Could you check a few things on this model? Use its own coordinates, in mm. A direction names the side the tool comes from. Round coordinates to 2 decimals unless told otherwise and drop trailing zeros. Write each loop counter-clockwise with the first axis right and the second up, starting at its lowest first coordinate (ties: lowest second). Pieces come first, ordered by that corner, then holes. Notation, with made-up numbers: M 12,73 L 20,73 A23 cw 20,108 Z; hole C 53,-36.75 d8. An arc over 180 degrees is marked long. One line per item, written item: value. Start each with the question number.
(1) I'm going to push a flat-ended pin straight in: pin 1 Ø6 at (x, z) = (12.5, 54) entering from +Y. Where does the tip first touch, or does it pass through?
(2) Thinking about a two-plate mould opening in Z: for faces 4 (the face through (21, 0, 37)), 5 (the face through (21, -3, 72)), 6 (the face through (5, -3, 25)), which applies, released by +Z, released by -Z, zero draft, split by the parting line, or undercut?
(3) If I drill on L1, parallel to Z at x = 21, y = -3.3; L2, parallel to X at y = -3.1, z = 6; L3, parallel to Z at x = 40.5, y = -3.45, over which ranges is the centre line in solid material (lowest first)?
(4) I want a section at B-B on y = -2.2. Please give me the cut outline in (x, z).
(5) I want a section at A-A on x = 39.5. Please give me the cut outline in (y, z).
(6) Which directions (+Z, -Z, +X, -X, +Y, -Y) give clear straight access to the entire face, cutting with the end or side of a thin tool? Please do faces 1 (the face through (39, -3, 29.584)), 2 (the face through (21, -3, 0)), 3 (the face through (2, -3, 27.498)).
```python
from build123d import *

# Parameters (mm, degrees)
F1_DEPTH = 6


with BuildPart() as f1:
    # F0 (on Front) → F1 (new body)
    with BuildSketch(Plane.XZ):
        Polygon((0, 22.498155), (0, 0), (42, 0), (42, 24.584079), (37, 24.584079), (37, 29.584079), (42, 29.584079), (42, 72), (0, 72), (0, 51), (0, 33.329517), (0, 27.498155), (5, 27.498155), (5, 22.498155), align=None)
        with BuildLine():
            ThreePointArc((22.5, 6), (19.93934, 4.93934), (21, 7.5))
            ThreePointArc((21, 7.5), (22.06066, 7.06066), (22.5, 6))
        make_face(mode=Mode.SUBTRACT)
        with BuildLine():
            ThreePointArc((21, 19.5), (19.5, 21), (21, 22.5))
            ThreePointArc((21, 22.5), (22.06066, 22.06066), (22.5, 21))
            ThreePointArc((22.5, 21), (22.06066, 19.93934), (21, 19.5))
        make_face(mode=Mode.SUBTRACT)
        with BuildLine():
            ThreePointArc((21, 49.5), (19.93934, 49.93934), (19.5, 51))
            ThreePointArc((19.5, 51), (21, 52.5), (22.5, 51))
            ThreePointArc((22.5, 51), (22.06066, 49.93934), (21, 49.5))
        make_face(mode=Mode.SUBTRACT)
    extrude(amount=F1_DEPTH)


solid = f1.part
```
Found:
1. pin 1: stops at y = 0
2. face 4: zero draft
2. face 5: released by +Z
2. face 6: undercut
3. L1: z = 0 to 4.5, 7.5 to 19.5, 22.5 to 49.5, 52.5 to 72
3. L2: x = 0 to 19.5, 22.5 to 42
3. L3: z = 0 to 24.58, 29.58 to 72
4. outline: M 0,0 L 42,0 L 42,24.58 L 37,24.58 L 37,29.58 L 42,29.58 L 42,72 L 0,72 L 0,27.5 L 5,27.5 L 5,22.5 L 0,22.5 Z; hole C 21,6 d3; hole C 21,21 d3; hole M 19.5,51 A1.5 ccw 21,49.5 A1.5 ccw long Z
5. outline: M -6,0 L 0,0 L 0,24.58 L -6,24.58 Z; M -6,29.58 L 0,29.58 L 0,72 L -6,72 Z
6. face 1: +X, +Y, -Y
6. face 2: -Z, +X, -X, +Y, -Y
6. face 3: -X, +Y, -Y
